Read the model definition and answer for the solid it produces. Units are mm, in the model's axes. A direction names the side the tool comes from. Give positions to 0.01 mm unless a question says otherwise; leave off trailing zeros. Write each loop counter-clockwise with the first axis right and the second up, starting at its lowest first coordinate (ties: lowest second). Pieces come first, ordered by that corner, then holes. Notation, with made-up numbers: (75, 70) -> (92, 70) arc R21 cw to (92, 82) -> close; hole circle Ø9 at (-17, 82). An arc over 180 degrees is marked (long way). Write item = value, one per line.
from build123d import *

# Parameters (mm, degrees)
F0_W          = 10.0419273615
F0_H          = 2.1
F0_H_2        = 6.8497342706
F1_DEPTH      = 25
F3_DEPTH      = 10
F3_DEPTH_BACK = 35
F4_W          = 7
F4_H          = 20.8
F5_DEPTH      = 10.0429273615
F6_R          = 1.25
F7_DEPTH      = 25
F8_R          = 5
F9_R          = 3


with BuildPart() as f1:
    # F0 (on Top) → F1 (new body)
    with BuildSketch(Plane.XY):
        with Locations((14.1209636807, 1.05)):
            Rectangle(F0_W, F0_H)
        with Locations((14.1209636807, 5.5248671353)):
            Rectangle(F0_W, F0_H_2)
    extrude(amount=F1_DEPTH)

    # F0 (on Top) → F3 (join, two sides)
    with BuildSketch(Plane.XY) as f3_sk:
        with Locations((14.1209636807, 1.05)):
            Rectangle(F0_W, F0_H)
    extrude(amount=-F3_DEPTH)
    extrude(f3_sk.sketch, amount=F3_DEPTH_BACK)

    # F4 (on offset) → F5 (cut, through all)
    with BuildSketch(Plane.YZ.offset(19.1419273615)):
        with Locations((3.5, 12.5)):
            Rectangle(F4_W, F4_H)
    extrude(amount=-F5_DEPTH, mode=Mode.SUBTRACT)

    # F6 (on Front) → F7 (cut)
    with BuildSketch(Plane.XZ):
        with Locations((14.1, 30)):
            Circle(F6_R)
        with Locations((14.1, -5)):
            Circle(F6_R)
    extrude(amount=-F7_DEPTH, mode=Mode.SUBTRACT)

    # F8
    f8_edges = [f1.edges().sort_by_distance(p)[0] for p in [
        (19.141927, 1.05, 35),
        (9.1, 1.05, 35),
        (9.1, 1.05, -10),
        (19.141927, 1.05, -10),
        (14.120964, 7, 2.1),
        (14.120964, 7, 22.9),
        (14.120964, 8.949734, 0),
        (14.120964, 8.949734, 25),
    ]]
    fillet(f8_edges, radius=F8_R)

    # F9
    f9_edges = [f1.edges().sort_by_distance(p)[0] for p in [
        (14.120964, 2.1, 0),
        (14.120964, 2.1, 25),
    ]]
    fillet(f9_edges, radius=F9_R)


solid = f1.part
(1) For a pull along Z with two mould halves and no side action, classify faces 1 (the flat face through (14, 8.95, 12)), 2 (the cylindrical face through (17.64, 1.06, 33.57)), 3 (the cylindrical face through (13.11, 1.04, -5.76)), 4 (the cylindrical face through (14.191, 7.763, 1.766)) as released by +Z, released by -Z, zero draft, split by the parting line, or undercut.
Checks:
face_1 = zero draft
face_2 = released by +Z
face_3 = undercut
face_4 = released by -Z
(2) A tool of negligible diameter and unlimited length cuts with its end or side. For faces 5 (the flat face through (9.1, 7.4, 12.6)), 6 (the flat face through (14.1, 2.1, -6.4)), 7 (the flat face through (14.05, 2.1, 31.41)), 8 (the flat face through (19.142, 7.4, 12.6)), 9 (the cylindrical face through (14.05, 5.5, 3.53)), from which of +Z, -Z, +X, -X, +Y, -Y can it reach the whole face along a straight path? Write none if from no direction.
Checks:
face_5 = +Z, -Z, -X, +Y, -Y
face_6 = -Z, +X, -X, +Y
face_7 = +Z, +X, -X, +Y
face_8 = +Z, -Z, +X, +Y, -Y
face_9 = +X, -X, -Y
(3) The part is cut by section B-B on z = 7.5. Determine the outline of the cut face in (x, y), plus the area to 3 significant figures.
Checks:
outline = (9.1, 7) -> (19.14, 7) -> (19.14, 8.95) -> (9.1, 8.95) -> close
area = 19.6 mm²
(4) The part is cut by section A-A on y = 5.5. Determine the outline of the cut face in (x, z), plus the area to 3 significant figures.
Checks:
outline = (9.1, 0.25) -> (19.14, 0.25) -> (19.14, 3.53) -> (9.1, 3.53) -> close; (9.1, 21.47) -> (19.14, 21.47) -> (19.14, 24.75) -> (9.1, 24.75) -> close
area = 65.9 mm²
(5) The part is cut by section D-D on y = 8.5. Determine the outline of the cut face in (x, z), plus the area to 3 significant figures.
Checks:
outline = (9.1, 2.93) -> (19.14, 2.93) -> (19.14, 22.07) -> (9.1, 22.07) -> close
area = 192 mm²
(6) Consider L1, parallel to Z at x = 14.1, y = 1.2; L2, parallel to Y at x = 18.5, z = 16; L3, parallel to Y at x = 17.25, z = 31. Determine where each line is inside the solid, lowest interval first.
Checks:
L1 = -10 to -6.25, -3.75 to 2.1, 22.9 to 28.75, 31.25 to 35
L2 = 7 to 8.95
L3 = 0 to 2.1
(7) The part is cut by section C-C on x = 13.25. Count the separate pieces of the cut face and the enclosed holes in it, plus the area to 3 significant figures.
Checks:
separate_pieces = 3
enclosed_holes = 0
area = 116 mm²
(8) Given P1, Ø2, axis at x = 16.5, y = 1.5, coming from the +Z side; P2, Ø2, axis at x = 11.5, z = 25, coming from the +Y side; P3, Ø5.5, axis at x = 16.5, z = -7.5, coming from the +Y side; P4, Ø1.5, axis at x = 14.1, z = -5, coming from the -Y side, each flat-ended and moving along its own axis, determine where each tip first touches the part or whether it passes through.
Checks:
P1 = 34.81
P2 = 6.95
P3 = 2.1
P4 = through
